Verification items for the finished model (mm, model axes). A direction names the side the tool comes from. Round coordinates to 2 decimals unless told otherwise and drop trailing zeros. Loops run counter-clockwise (first coordinate to the right, second up) from the corner with the lowest first, then second, coordinate; pieces in that order, holes last. Notation, with made-up numbers: (89, -3.75) -> (127, -3.75) arc R22 cw to (127, 22.25) -> close; hole circle Ø2 at (79, 64.25). An arc over 180 degrees is marked (long way). Write item = value, one per line.
```python
from build123d import *

# Parameters (mm, degrees)
SKETCH2_R          = 1.25
CUT_EXTRUDE1_DEPTH = 33.687229922
SKETCH3_R          = 2.5
CUT_EXTRUDE2_DEPTH = 16.5
SKETCH7_R          = 4.725
CUT_EXTRUDE7_DEPTH = 10
FILLET1_R          = 2
SKETCH8_RX         = 3
SKETCH8_RY         = 1.5
CUT_EXTRUDE8_DEPTH = 2.5
SKETCH4_R          = 1.25
CUT_EXTRUDE5_DEPTH = 5


with BuildPart() as part:
    # Sketch1 → Revolve1 (revolve)
    with BuildSketch(Plane(origin=(0, 0, 0), x_dir=(1, 0, 0), z_dir=(0, 1, 0)), mode=Mode.PRIVATE) as revolve1_sk:
        Polygon((12.139813159, 7), (12.139813159, 12.05), (9.139813159, 15.55), (10.139813159, 15.55), (10.139813159, 16.55), (10.139813159, 18.55), (8.639813159, 18.55), (8.639813159, 16.55), (-7.360186841, 16.55), (-7.360186841, 14.55), (-7.360186841, 0), (11.541615212, 0), (11.541615212, 5.071775549), (10.139813159, 5.071775549), (10.139813159, 5.571775549), align=None)
    revolve(revolve1_sk.sketch.rotate(Axis((-37.278866169, 0, 0), (1, 0, 0)), 180), axis=Axis((-37.278866169, 0, 0), (1, 0, 0)))

    # Sketch2 → Cut-Extrude1 (cut, through all)
    with BuildSketch(Plane(origin=(12.139813159, 0, 0), x_dir=(0, 0, -1), z_dir=(1, 0, 0))):
        with Locations((0, 10)):
            Circle(SKETCH2_R)
        with Locations((7.071067812, 7.071067812)):
            Circle(SKETCH2_R)
        with Locations((10, 0)):
            Circle(SKETCH2_R)
        with Locations((7.071067812, -7.071067812)):
            Circle(SKETCH2_R)
        with Locations((0, -10)):
            Circle(SKETCH2_R)
        with Locations((-7.071067812, -7.071067812)):
            Circle(SKETCH2_R)
        with Locations((-10, 0)):
            Circle(SKETCH2_R)
        with Locations((-7.071067812, 7.071067812)):
            Circle(SKETCH2_R)
    extrude(amount=-CUT_EXTRUDE1_DEPTH, mode=Mode.SUBTRACT)

    # Sketch3 → Cut-Extrude2 (cut)
    with BuildSketch(Plane.ZY.offset(7.360186841)):
        with Locations((0, 10)):
            Circle(SKETCH3_R)
        with Locations((7.071067812, 7.071067812)):
            Circle(SKETCH3_R)
        with Locations((10, 0)):
            Circle(SKETCH3_R)
        with Locations((7.071067812, -7.071067812)):
            Circle(SKETCH3_R)
        with Locations((0, -10)):
            Circle(SKETCH3_R)
        with Locations((-7.071067812, -7.071067812)):
            Circle(SKETCH3_R)
        with Locations((-10, 0)):
            Circle(SKETCH3_R)
        with Locations((-7.071067812, 7.071067812)):
            Circle(SKETCH3_R)
    extrude(amount=-CUT_EXTRUDE2_DEPTH, mode=Mode.SUBTRACT)

    # Sketch7 → Cut-Extrude7 (cut)
    with BuildSketch(Plane.ZY.offset(7.360186841)):
        Circle(SKETCH7_R)
    extrude(amount=-CUT_EXTRUDE7_DEPTH, mode=Mode.SUBTRACT)

    # Fillet1
    # the kernel refuses this fillet: 2 mm, written as the material it takes off along each edge
    with BuildSketch(Plane(origin=(11.541615212, 0, 0), x_dir=(0, 0, 1), z_dir=(0, 1, 0))) as fillet1_piece_1:
        with BuildLine():
            CenterArc((3.163331362, -2), FILLET1_R, 17.403493434, 72.596506566)
            Line((3.163331362, 0), (3.163331362, 0.04))
            Line((3.163331362, 0.04), (5.071775549, 0.04))
            Line((5.071775549, 0.04), (5.111775549, 0))
            ThreePointArc((5.111775549, 0), (5.111775549, -0.700901026), (5.109944433, -1.389838094))
            Line((5.109944433, -1.389838094), (5.071775549, -1.401802053))
        make_face()
    revolve(axis=Axis((11.541615212, 0, 0), (1, 0, 0)), mode=Mode.SUBTRACT)

    # Sketch8 → Cut-Extrude8 (cut, symmetric)
    with BuildSketch(Plane(origin=(10.139813159, 0, 0), x_dir=(0, 0, -1), z_dir=(1, 0, 0))):
        with Locations((0, 13.8)):
            Ellipse(SKETCH8_RX, SKETCH8_RY)
        with Locations(Location((11.951150572, 6.9), (0, 0, 120))):
            Ellipse(SKETCH8_RX, SKETCH8_RY)
        with Locations(Location((11.951150572, -6.9), (0, 0, -120))):
            Ellipse(SKETCH8_RX, SKETCH8_RY)
        with Locations(Location((0, -13.8), (0, 0, 180))):
            Ellipse(SKETCH8_RX, SKETCH8_RY)
        with Locations(Location((-11.951150572, -6.9), (0, 0, 120))):
            Ellipse(SKETCH8_RX, SKETCH8_RY)
        with Locations(Location((-11.951150572, 6.9), (0, 0, -120))):
            Ellipse(SKETCH8_RX, SKETCH8_RY)
    extrude(amount=CUT_EXTRUDE8_DEPTH, both=True, mode=Mode.SUBTRACT)

    # Sketch4 → Cut-Extrude5 (cut)
    with BuildSketch(Plane(origin=(13.139813159, 0, 0), x_dir=(0, 0, -1), z_dir=(1, 0, 0))):
        with Locations((0, 13.75)):
            Circle(SKETCH4_R)
    extrude(amount=-CUT_EXTRUDE5_DEPTH, mode=Mode.SUBTRACT)


solid = part.part
```
(1) Material ranges on probe 1 along Y at (x, z) = (9.65, 0); probe 2 along Y at (x, z) = (10.75, 0); probe 3 along Y at (x, z) = (0.5, 0.5), recorded low to high. Write a range as from..to.
Filled sheet:
probe_1 = -18.55..-15.55, -12.3..-11.25, -8.75..8.75, 11.25..12.3, 15.55..18.55
probe_2 = -12.3..-11.25, -8.75..-6.01, -4.76..4.76, 6.01..8.75, 11.25..12.3
probe_3 = -16.54..-12.45, -7.55..-4.7, 4.7..7.55, 12.45..16.54
(2) Sectioned sample at A-A, the plane z = 16. Record the cut outline in (x, y), and give its area (3 significant figures).
Filled sheet:
outline = (-7.36, -4.23) -> (8.64, -4.23) -> (8.64, -9.39) -> (10.14, -9.39) -> (10.14, 9.39) -> (8.64, 9.39) -> (8.64, 4.23) -> (-7.36, 4.23) -> close
area = 164 mm2
(3) Set-up check for faces 1 (the face through (-7.36, 3.45, 3.45)), 2 (the face through (0.8, 0.1, 7.5)), 3 (the face through (7.64, 7, 12)): record each of +Z, -Z, +X, -X, +Y, -Y from which the full face is reachable in a straight line by a thin tool's end or side.
Filled sheet:
face_1 = +Z, -Z, -X, +Y, -Y
face_2 = -X
face_3 = +X
(4) Go/stop test with flat-tipped pins: pin 1 Ø6 at (y, z) = (9, 1) entering from -X; pin 2 Ø3 at (y, z) = (-1.5, -0.5) entering from +X; pin 3 Ø2 at (x, y) = (-1.5, -10) entering from +Z; pin 4 Ø1 at (x, z) = (-1.5, 4) entering from +Y. Record where each tip stops, or that it passes through.
Filled sheet:
pin_1 = -7.36
pin_2 = 11.54
pin_3 = 13.89
pin_4 = 16.18
(5) Draft check along Z on faces 4 (the face through (2.64, 0, 0)), 5 (the face through (10.14, 9.5, 12.5)). Enter one of: released by +Z, released by -Z, zero draft, split by the parting line, or undercut.
Filled sheet:
face_4 = undercut
face_5 = zero draft
(6) Sectioned sample at B-B, the plane x = 5. Count the separate pieces of the cut face and the enclosed holes in it, and give its area (3 significant figures).
Filled sheet:
separate_pieces = 1
enclosed_holes = 8
area = 703 mm2
